Geometry check sheet. Reference: the model listing, model coordinates, mm. A direction names the side the tool comes from. Coordinates: 2 decimals unless noted, no trailing zeros. Loops run counter-clockwise (first coordinate to the right, second up) from the corner with the lowest first, then second, coordinate; pieces in that order, holes last. Notation, with made-up numbers: (0, 61) - (39, 61) arc R12 ccw to (39, 68) - close; hole circle Ø2 at (-1, 69.25). An arc over 180 degrees is marked (long way). One line per item, written item: value.
from build123d import *

# Parameters (mm, degrees)
SKETCH_1_R      = 5.25
SKETCH_1_R_2    = 1.65
EXTRUDE_1_DEPTH = 3.3
FILLET_1_R      = 10


with BuildPart() as part:
    # 草图1 → 凸台-拉伸1 (new body)
    with BuildSketch(Plane.XY):
        Polygon((-27.25, -3.25), (-27.25, 18.75), (-2.25, 18.75), (-2.25, 40.25), (17.75, 40.25), (17.75, 18.75), (42.75, 18.75), (42.75, -3.25), (17.75, -3.25), (17.75, -24.75), (-2.25, -24.75), (-2.25, -3.25), align=None)
        with Locations((34.75, 7.75)):
            Circle(SKETCH_1_R, mode=Mode.SUBTRACT)
        with Locations((-19.25, 7.75)):
            Circle(SKETCH_1_R, mode=Mode.SUBTRACT)
        with Locations((7.75, 33.25)):
            Circle(SKETCH_1_R_2, mode=Mode.SUBTRACT)
        with Locations((7.75, -18.25)):
            Circle(SKETCH_1_R_2, mode=Mode.SUBTRACT)
        with BuildLine():
            Line((4.258939989, 0), (11.241060011, 0))
            ThreePointArc((11.241060011, 0), (13.76040764, 1.73959236), (15.5, 4.258939989))
            Line((15.5, 4.258939989), (15.5, 11.241060011))
            ThreePointArc((15.5, 11.241060011), (13.76040764, 13.76040764), (11.241060011, 15.5))
            Line((11.241060011, 15.5), (4.258939989, 15.5))
            ThreePointArc((4.258939989, 15.5), (1.73959236, 13.76040764), (0, 11.241060011))
            Line((0, 11.241060011), (0, 4.258939989))
            ThreePointArc((0, 4.258939989), (1.73959236, 1.73959236), (4.258939989, 0))
        make_face(mode=Mode.SUBTRACT)
    extrude(amount=EXTRUDE_1_DEPTH)

    # 圆角1
    fillet_1_edges = [part.edges().sort_by_distance(p)[0] for p in [
        (-27.25, 18.75, 1.65),
        (-27.25, -3.25, 1.65),
        (-2.25, -3.25, 1.65),
        (-2.25, -24.75, 1.65),
        (17.75, -24.75, 1.65),
        (17.75, -3.25, 1.65),
        (42.75, -3.25, 1.65),
        (42.75, 18.75, 1.65),
        (17.75, 18.75, 1.65),
        (-2.25, 18.75, 1.65),
        (-2.25, 40.25, 1.65),
        (17.75, 40.25, 1.65),
    ]]
    fillet(fillet_1_edges, radius=FILLET_1_R - 0.0001)  # a hair under: the kernel refuses the full size


solid = part.part
(1) Access from +Z, -Z, +X, -X, +Y, -Y to the whole of each face (thin tool, end or side, straight path). Record for faces 1 (the face through (1.71, 1.77, 1.63)), 2 (the face through (-15, -3.25, 2)), 3 (the face through (-15, 18.75, 2)), 4 (the face through (30, -3.25, 2)).
Reply:
face 1: +Z, -Z
face 2: +Z, -Z, -X, -Y
face 3: +Z, -Z, -X, +Y
face 4: +Z, -Z, +X, -Y
(2) Release check for a two-part mould opening along Y. For faces 5 (the face through (0.6, -21.74, 1.67)), 6 (the face through (17.75, -14, 2)), 7 (the face through (8, 0, 2)) record: pulls with the +Y half, pulls with the -Y half, needs draft (parallel to the pull), parting line crosses it, or undercut.
Reply:
face 5: pulls with the -Y half
face 6: needs draft
face 7: undercut
(3) Cross-section at D-D on z = 1.3. State how many separate pieces and enclosed holes the cut face has, and give its area (3 significant figures).
Reply:
separate pieces: 1
enclosed holes: 5
area: 1,910 mm2
(4) Cross-section at B-B on y = -18.25. Record the cut outline in (x, z).
Reply:
outline: (-1.62, 0) - (6.1, 0) - (6.1, 3.3) - (-1.62, 3.3) - close; (9.4, 0) - (17.12, 0) - (17.12, 3.3) - (9.4, 3.3) - close
(5) Go/stop test with flat-tipped pins: pin 1 Ø1.6 at (x, z) = (9.5, 1.5) entering from +Y; pin 2 Ø0.5 at (y, z) = (29.5, 1) entering from -X; pin 3 Ø1 at (x, y) = (33.5, 4) entering from +Z; pin 4 Ø0.5 at (y, z) = (-13.5, 2.5) entering from +X. Record where each tip stops, or that it passes through.
Reply:
pin 1: y = 40.2
pin 2: x = -2.25
pin 3: through
pin 4: x = 17.75
(6) Cross-section at A-A on y = 7.75. Record the cut outline in (x, z), and give its area (3 significant figures).
Reply:
outline: (-27.25, 0) - (-24.5, 0) - (-24.5, 3.3) - (-27.25, 3.3) - close; (-14, 0) - (0, 0) - (0, 3.3) - (-14, 3.3) - close; (15.5, 0) - (29.5, 0) - (29.5, 3.3) - (15.5, 3.3) - close; (40, 0) - (42.75, 0) - (42.75, 3.3) - (40, 3.3) - close
area: 111 mm2
(7) Cross-section at C-C on x = 2. Record the cut outline in (y, z).
Reply:
outline: (-22.93, 0) - (1.49, 0) - (1.49, 3.3) - (-22.93, 3.3) - close; (14.01, 0) - (38.43, 0) - (38.43, 3.3) - (14.01, 3.3) - close
(8) Material ranges on probe 1 along X at (y, z) = (8, 0.2); probe 2 along X at (y, z) = (10.5, 2.95); probe 3 along X at (y, z) = (-15, 0.15), recorded low to high. Write a range as from..to.
Reply:
probe 1: -27.25..-24.49, -14.01..0, 15.5..29.51, 39.99..42.75
probe 2: -27.1..-23.72, -14.78..0, 15.5..30.28, 39.22..42.6
probe 3: -2.25..17.75
